```python
from build123d import *

# Parameters (mm, degrees)
MOUNT_BASE_DEPTH               = 10
SKETCH_8_W                     = 38
SKETCH_8_H                     = 31
CUT_BASE_DEPTH                 = 34
SKETCH10_W                     = 3
SKETCH10_H                     = 31
BEND_SIDES_DEPTH               = 34.2
SKETCH16_W                     = 44
SKETCH16_H                     = 3
WIRE_SIDES_DEPTH               = 34.2
DRAFT9_ANGLE                   = 1
DRAFT10_ANGLE                  = 1
DIFFERENTIAL_CLAMP_DEPTH       = 10
DIFFERENTIAL_CLAMP_DEPTH_BACK  = 8.6
DIFFERENTIAL_BAR_CUT_DEPTH     = 3.6
STRUCTURAL_SCREW_W_HEADS_DEPTH = 5
SKETCH25_R                     = 1.7
SCREW_HOLES_DEPTH              = 24
NUT_HOLE_DEPTH                 = 2.6
FILLET7_R                      = 2
FILLET8_R                      = 2
FILLET9_R                      = 2
FILLET10_R                     = 2
FILLET15_R                     = 2
BOSS_EXTRUDE1_DEPTH            = 17.6
CUT_EXTRUDE6_DEPTH             = 8.6
SKETCH48_W                     = 74
SKETCH48_H                     = 70
CUT_EXTRUDE9_DEPTH             = 17.6
SKETCH49_W                     = 77
SKETCH49_H                     = 70
BOSS_EXTRUDE2_DEPTH            = 1
SKETCH50_R                     = 1.7
CUT_EXTRUDE10_DEPTH            = 1
CUT_EXTRUDE12_DEPTH            = 34.2
SKETCH53_W                     = 19
SKETCH53_H                     = 5.77151387
CUT_EXTRUDE13_DEPTH            = 30
FILLET17_R                     = 2
BOSS_EXTRUDE3_DEPTH            = 34.2
CUT_EXTRUDE14_DEPTH            = 2.6
SKETCH56_R                     = 1.7
CUT_EXTRUDE15_DEPTH            = 8
FILLET18_R                     = 2
FILLET20_R                     = 0.5


with BuildPart() as part:
    # Sketch6 → Mount Base (new body)
    with BuildSketch(Plane(origin=(0, 0, 0), x_dir=(0, 1, 0), z_dir=(0, 0, 1))):
        Polygon((-30, -26.5), (-30, -31.5), (30, -31.5), (30, -26.5), (30, 26.5), (-30, 26.5), align=None)
    extrude(amount=MOUNT_BASE_DEPTH)

    # Sketch 8 → Cut-Base (cut)
    with BuildSketch(Plane(origin=(0, 0, 7), x_dir=(0, 1, 0), z_dir=(0, 0, 1))):
        Rectangle(SKETCH_8_W, SKETCH_8_H)
    extrude(amount=CUT_BASE_DEPTH, mode=Mode.SUBTRACT)

    # Sketch10 → Bend Sides (add)
    with BuildSketch(Plane(origin=(0, 0, 10), x_dir=(0, 1, 0), z_dir=(0, 0, 1))):
        with Locations((-20.5, 0)):
            Rectangle(SKETCH10_W, SKETCH10_H)
        with Locations((20.5, 0)):
            Rectangle(SKETCH10_W, SKETCH10_H)
    extrude(amount=BEND_SIDES_DEPTH)

    # Sketch16 → Wire Sides (add)
    with BuildSketch(Plane(origin=(0, 0, 10), x_dir=(0, 1, 0), z_dir=(0, 0, 1))):
        with Locations((0, -17)):
            Rectangle(SKETCH16_W, SKETCH16_H)
        with Locations((0, 17)):
            Rectangle(SKETCH16_W, SKETCH16_H)
    extrude(amount=WIRE_SIDES_DEPTH)

    # Draft9
    draft9_faces = [part.faces().sort_by_distance(p)[0] for p in [
        (0, -19, 25.6),
    ]]
    draft(draft9_faces, Plane(origin=(0, 0, 0), x_dir=(-1, 0, 0), z_dir=(0, 0, -1)), DRAFT9_ANGLE)

    # Draft10
    draft10_faces = [part.faces().sort_by_distance(p)[0] for p in [
        (0, 19, 25.6),
    ]]
    draft(draft10_faces, Plane(origin=(0, 0, 0), x_dir=(-1, 0, 0), z_dir=(0, 0, -1)), DRAFT10_ANGLE)

    # Sketch20 → Differential Clamp (add, two sides)
    with BuildSketch(Plane(origin=(0, 0, 0), x_dir=(0, 1, 0), z_dir=(0, 0, 1))) as differential_clamp_sk:
        Polygon((-30, 37), (-30, 26.5), (-30, -37), (30, -37), (30, 27), (30, 37), align=None)
    extrude(amount=DIFFERENTIAL_CLAMP_DEPTH)
    extrude(differential_clamp_sk.sketch, amount=-DIFFERENTIAL_CLAMP_DEPTH_BACK)

    # Sketch22 → Differential Bar cut (cut)
    with BuildSketch(Plane(origin=(0, 0, 0), x_dir=(0, 1, 0), z_dir=(0, 0, 1))):
        Polygon((-86.956180584, -24.693764348), (0, -30.5), (86.956180584, -24.693764348), (86.956180584, 37), (30, 37), (-30, 37), (-86.956180584, 37), align=None)
    extrude(amount=-DIFFERENTIAL_BAR_CUT_DEPTH, mode=Mode.SUBTRACT)

    # Sketch 7 → Structural Screw w/ heads (cut)
    with BuildSketch(Plane(origin=(0, 0, 0), x_dir=(0, 1, 0), z_dir=(0, 0, 1))):
        with BuildLine():
            Line((-22.42, 37.163783556), (-22.42, -19.42))
            ThreePointArc((-22.42, -19.42), (-19.42, -22.42), (-16.42, -19.42))
            Line((-16.42, -19.42), (-16.42, 37.163783556))
            Line((-16.42, 37.163783556), (-22.42, 37.163783556))
        make_face()
        with BuildLine():
            Line((16.42, -19.42), (16.42, 37.161181528))
            Line((16.42, 37.161181528), (22.42, 37.161181528))
            Line((22.42, 37.161181528), (22.42, -19.42))
            ThreePointArc((22.42, -19.42), (19.42, -22.42), (16.42, -19.42))
        make_face()
        with BuildLine():
            Line((-3, 37.161181528), (3, 37.161181528))
            Line((3, 37.161181528), (3, -10.32))
            ThreePointArc((3, -10.32), (0, -13.32), (-3, -10.32))
            Line((-3, -10.32), (-3, 37.161181528))
        make_face()
    extrude(amount=STRUCTURAL_SCREW_W_HEADS_DEPTH, mode=Mode.SUBTRACT)

    # Sketch25 → Screw holes (cut)
    with BuildSketch(Plane.XY.offset(10)):
        with Locations((-32, 29)):
            Circle(SKETCH25_R)
        with Locations((-32, -29)):
            Circle(SKETCH25_R)
        with Locations((32, -29)):
            Circle(SKETCH25_R)
        with Locations((32, 29)):
            Circle(SKETCH25_R)
    extrude(amount=-SCREW_HOLES_DEPTH, mode=Mode.SUBTRACT)

    # Sketch27 → Nut hole (cut)
    with BuildSketch(Plane(origin=(0, 0, -8.6), x_dir=(-1, 0, 0), z_dir=(0, 0, -1))):
        Polygon((31.935113153, 25.709743217), (34.817002535, 27.29867795), (34.881889383, 30.588934733), (32.064886847, 32.290256783), (29.182997465, 30.70132205), (29.118110617, 27.411065267), align=None)
        Polygon((28.709103466, -29), (30.354551733, -31.85), (33.645448267, -31.85), (35.290896534, -29), (33.645448267, -26.15), (30.354551733, -26.15), align=None)
        Polygon((-30.354551733, -26.15), (-28.709103466, -29), (-30.354551733, -31.85), (-33.645448267, -31.85), (-35.290896534, -29), (-33.645448267, -26.15), align=None)
        Polygon((-29.118110617, 27.411065267), (-31.935113153, 25.709743217), (-34.817002535, 27.29867795), (-34.881889383, 30.588934733), (-32.064886847, 32.290256783), (-29.182997465, 30.70132205), align=None)
    extrude(amount=-NUT_HOLE_DEPTH, mode=Mode.SUBTRACT)

    # Fillet7
    fillet7_edges = [part.edges().sort_by_distance(p)[0] for p in [
        (-37, 30, 5),
    ]]
    fillet(fillet7_edges, radius=FILLET7_R)

    # Fillet8
    fillet8_edges = [part.edges().sort_by_distance(p)[0] for p in [
        (-37, -30, 5),
    ]]
    fillet(fillet8_edges, radius=FILLET8_R)

    # Fillet9
    fillet9_edges = [part.edges().sort_by_distance(p)[0] for p in [
        (-37, 30, -6.1),
    ]]
    fillet(fillet9_edges, radius=FILLET9_R)

    # Fillet10
    fillet10_edges = [part.edges().sort_by_distance(p)[0] for p in [
        (-37, -30, -6.1),
    ]]
    fillet(fillet10_edges, radius=FILLET10_R)

    # Fillet15
    fillet15_edges = [part.edges().sort_by_distance(p)[0] for p in [
        (0, 18.825449351, 10),
        (0, -18.825449351, 10),
    ]]
    fillet(fillet15_edges, radius=FILLET15_R)

    # Sketch42 → Boss-Extrude1 (add)
    with BuildSketch(Plane.XY.offset(-8.6)):
        Polygon((37, 35), (-37, 35), (-37, 23), (28.5, 23), (28.5, -23), (-37, -23), (-37, -35), (37, -35), align=None)
    extrude(amount=BOSS_EXTRUDE1_DEPTH)

    # Sketch43 → Cut-Extrude6 (cut)
    with BuildSketch(Plane(origin=(0, 0, 0), x_dir=(-1, 0, 0), z_dir=(0, 0, -1))):
        Polygon((-24.693764348, 86.956180584), (37, 86.956180584), (37, -86.956180584), (-24.693764348, -86.956180584), (-30.5, 0), align=None)
    extrude(amount=CUT_EXTRUDE6_DEPTH, mode=Mode.SUBTRACT)

    # Sketch48 → Cut-Extrude9 (cut)
    with BuildSketch(Plane.XY.offset(9)):
        Rectangle(SKETCH48_W, SKETCH48_H)
    extrude(amount=-CUT_EXTRUDE9_DEPTH, mode=Mode.SUBTRACT)

    # Sketch49 → Boss-Extrude2 (add)
    with BuildSketch(Plane.XY.offset(9)):
        Rectangle(SKETCH49_W, SKETCH49_H)
    extrude(amount=BOSS_EXTRUDE2_DEPTH)

    # Sketch50 → Cut-Extrude10 (cut)
    with BuildSketch(Plane.XY.offset(9)):
        with Locations((-32.5, 29)):
            Circle(SKETCH50_R)
        with Locations((34.25, 29)):
            Circle(SKETCH50_R)
        with Locations((34.25, -29)):
            Circle(SKETCH50_R)
        with Locations((-32.5, -29)):
            Circle(SKETCH50_R)
    extrude(amount=CUT_EXTRUDE10_DEPTH, mode=Mode.SUBTRACT)

    # Sketch52 → Cut-Extrude12 (cut)
    with BuildSketch(Plane.XY.offset(44.2)):
        Polygon((-15.5, 24.22848613), (-9.5, 24.22848613), (-9.5, 18.22848613), (-9.5, 16.790234565), (-15.5, 16.790234565), (-15.5, 18.22848613), align=None)
        Polygon((15.5, 18.22848613), (15.5, 16.790234565), (9.5, 16.790234565), (9.5, 18.22848613), (9.5, 24.22848613), (15.5, 24.22848613), align=None)
        Polygon((15.5, -18.22848613), (15.5, -24.22848613), (9.5, -24.22848613), (9.5, -18.22848613), (9.5, -16.790234565), (15.5, -16.790234565), align=None)
        Polygon((-15.5, -18.22848613), (-15.5, -16.790234565), (-9.5, -16.790234565), (-9.5, -18.22848613), (-9.5, -24.22848613), (-15.5, -24.22848613), align=None)
    extrude(amount=-CUT_EXTRUDE12_DEPTH, mode=Mode.SUBTRACT)

    # Sketch53 → Cut-Extrude13 (cut)
    with BuildSketch(Plane.XY.offset(44.2)):
        with Locations((0, -21.114243065)):
            Rectangle(SKETCH53_W, SKETCH53_H)
        with Locations((0, 19.114243065)):
            Rectangle(SKETCH53_W, SKETCH53_H)
    extrude(amount=-CUT_EXTRUDE13_DEPTH, mode=Mode.SUBTRACT)

    # Fillet17
    fillet17_edges = [part.edges().sort_by_distance(p)[0] for p in [
        (-9.5, -20.376069039, 14.2),
    ]]
    fillet(fillet17_edges, radius=FILLET17_R)

    # Sketch55 → Boss-Extrude3 (add)
    with BuildSketch(Plane.XY.offset(10)):
        Polygon((-18.5, 22), (-18.5, -22), (-15.5, -22), (-15.5, -25), (-27.5, -25), (-27.5, -22), (-27.5, 22), (-27.5, 25), (-15.5, 25), (-15.5, 22), align=None)
        Polygon((18.5, 22), (18.5, -22), (15.5, -22), (15.5, -25), (27.5, -25), (27.5, -22), (27.5, 22), (27.5, 25), (15.5, 25), (15.5, 22), align=None)
    extrude(amount=BOSS_EXTRUDE3_DEPTH)

    # Sketch54 → Cut-Extrude14 (cut)
    with BuildSketch(Plane.XY.offset(39.2)):
        Polygon((24.4, 20.359315781), (24.4, 17.010684219), (21.5, 15.336368439), (18.6, 17.010684219), (18.6, 20.359315781), (21.5, 22.033631561), align=None)
        Polygon((-24.4, 17.010684219), (-21.5, 15.336368439), (-18.6, 17.010684219), (-18.6, 20.359315781), (-21.5, 22.033631561), (-24.4, 20.359315781), align=None)
        Polygon((21.5, -22.033631561), (24.4, -20.359315781), (24.4, -17.010684219), (21.5, -15.336368439), (18.6, -17.010684219), (18.6, -20.359315781), align=None)
        Polygon((-24.4, -20.359315781), (-24.4, -17.010684219), (-21.5, -15.336368439), (-18.6, -17.010684219), (-18.6, -20.359315781), (-21.5, -22.033631561), align=None)
    extrude(amount=CUT_EXTRUDE14_DEPTH, mode=Mode.SUBTRACT)

    # Sketch56 → Cut-Extrude15 (cut)
    with BuildSketch(Plane.XY.offset(44.2)):
        with Locations((-21.5, 18.685)):
            Circle(SKETCH56_R)
        with Locations((21.5, 18.685)):
            Circle(SKETCH56_R)
        with Locations((21.5, -18.685)):
            Circle(SKETCH56_R)
        with Locations((-21.5, -18.685)):
            Circle(SKETCH56_R)
    extrude(amount=-CUT_EXTRUDE15_DEPTH, mode=Mode.SUBTRACT)

    # Fillet18
    fillet18_edges = [part.edges().sort_by_distance(p)[0] for p in [
        (9.5, -20.376069039, 14.2),
        (-9.5, 20.376069039, 14.2),
        (9.5, 20.376069039, 14.2),
        (-21.5, 25, 44.2),
        (-21.5, -25, 44.2),
        (21.5, -25, 44.2),
        (21.5, 25, 44.2),
    ]]
    fillet(fillet18_edges, radius=FILLET18_R)

    # Fillet20
    fillet20_edges = [part.edges().sort_by_distance(p)[0] for p in [
        (-27.5, 0, 44.2),
        (-27.5, -25, 26.1),
        (-27.5, 25, 26.1),
        (-27.5, -24.414213562, 43.614213562),
        (-27.5, 24.414213562, 43.614213562),
        (-15.5, 25, 26.1),
        (-15.5, -25, 26.1),
        (-15.5, -24.414213562, 43.614213562),
        (-15.5, 24.414213562, 43.614213562),
        (15.5, 0, 44.2),
        (27.5, 0, 44.2),
        (27.5, 25, 26.1),
        (27.5, -25, 26.1),
        (27.5, 24.414213562, 43.614213562),
        (27.5, -24.414213562, 43.614213562),
        (15.5, -25, 26.1),
        (15.5, 25, 26.1),
        (15.5, 24.414213562, 43.614213562),
        (15.5, -24.414213562, 43.614213562),
        (-15.5, 0, 44.2),
    ]]
    fillet(fillet20_edges, radius=FILLET20_R)


solid = part.part
```
Design review of the part built by this model. Coordinates are the model's own, in mm. A direction names the side the tool comes from. Round coordinates to 2 decimals unless told otherwise and drop trailing zeros. Order: outer loops, then holes, each group sorted by start corner. A loop starts at its lowest first (then second) coordinate and runs counter-clockwise, first axis right, second up. Notation, with made-up numbers: (52.5, 49) - (75.5, 49) arc R22 ccw to (75.5, 83) - close; hole circle Ø5 at (13.25, 53). An arc over 180 degrees is marked (long way). Return JSON: item names as keys, results as strings.
Q1. Consider section C-C on y = 11.5. Write out the cut boundary in (x, z).
Computed values:
{"outline": "(-38.5, 9) - (38.5, 9) - (38.5, 10) - (27.5, 10) - (27.5, 43.7) arc R0.5 ccw to (27, 44.2) - (16, 44.2) arc R0.5 ccw to (15.5, 43.7) - (15.5, 10) - (-15.5, 10) - (-15.5, 43.7) arc R0.5 ccw to (-16, 44.2) - (-27, 44.2) arc R0.5 ccw to (-27.5, 43.7) - (-27.5, 10) - (-38.5, 10) - close"}
Q2. For pin 1 Ø3 at (y, z) = (18, 40.5) entering from -X; pin 2 Ø3 at (x, z) = (17.5, 30) entering from -Y; pin 3 Ø1.6 at (x, y) = (-0.5, 21) entering from +Z, all flat-tipped, find the tip position at first contact; note any pin that passes through.
Computed values:
{"pin 1": "stops at x = -27.5", "pin 2": "stops at y = -25", "pin 3": "stops at z = 14.2"}
Q3. Machinability: for faces 4 (the flat face through (-9.5, 20, 11)), 5 (the flat face through (22.93, -21.21, 40.48)), 6 (the flat face through (-22, 19, 36.2)), which of the approach directions +Z, -Z, +X, -X, +Y, -Y give a long, thin tool a straight path to every point of the face, cutting with its end or side? Answer none if there is none.
Computed values:
{"face 4": "+Z, +Y, -Y", "face 5": "none", "face 6": "+Z"}
Q4. Consider section A-A on y = 29. Write out the cut boundary in (x, z).
Computed values:
{"outline": "(-38.5, 9) - (-34.2, 9) - (-34.2, 10) - (-38.5, 10) - close; (-30.8, 9) - (32.55, 9) - (32.55, 10) - (-30.8, 10) - close; (35.95, 9) - (38.5, 9) - (38.5, 10) - (35.95, 10) - close"}
Q5. Consider section B-B on z = 17. Write out the cut boundary in (x, y).
Computed values:
{"outline": "(-27.5, -24.5) arc R0.5 ccw to (-27, -25) - (-16, -25) arc R0.5 ccw to (-15.5, -24.5) - (-15.5, 24.5) arc R0.5 ccw to (-16, 25) - (-27, 25) arc R0.5 ccw to (-27.5, 24.5) - close; (15.5, -24.5) arc R0.5 ccw to (16, -25) - (27, -25) arc R0.5 ccw to (27.5, -24.5) - (27.5, 24.5) arc R0.5 ccw to (27, 25) - (16, 25) arc R0.5 ccw to (15.5, 24.5) - close"}
Q6. Consider section D-D on z = 11. Write out the cut boundary in (x, y), plus the area to 3 significant figures.
Computed values:
{"outline": "(-27.5, -24.5) arc R0.5 ccw to (-27, -25) - (-16, -25) arc R0.5 ccw to (-15.5, -24.5) - (-15.5, 24.5) arc R0.5 ccw to (-16, 25) - (-27, 25) arc R0.5 ccw to (-27.5, 24.5) - close; (-9.5, -22) - (9.5, -22) - (9.5, -18.52) - (-9.5, -18.52) - close; (-9.5, 18.52) - (9.5, 18.52) - (9.5, 22) - (-9.5, 22) - close; (15.5, -24.5) arc R0.5 ccw to (16, -25) - (27, -25) arc R0.5 ccw to (27.5, -24.5) - (27.5, 24.5) arc R0.5 ccw to (27, 25) - (16, 25) arc R0.5 ccw to (15.5, 24.5) - close", "area": "1,330 mm2"}
Q7. Wall thickness on L1, parallel to Y at x = -21.5, z = 38.65 (3 decimals); L2, parallel to Y at x = 21, z = 43; L3, parallel to X at y = 24, z = 41: over which ranges is each line inside the solid? List them lowest first. Write a range as [from, to].
Computed values:
{"L1": "y = [-25, -20.385], [-16.985, 16.985], [20.385, 25]", "L2": "y = [-24.83, -20.31], [-17.06, 17.06], [20.31, 24.83]", "L3": "x = [-27.5, -15.5], [15.5, 27.5]"}
Q8. The part is to be moulded in two halves that separate along Y. For faces 1 (the flat face through (-20.07, -16.16, 40.48)), 2 (the flat face through (0, 22, 12)), 3 (the flat face through (-21, -25, 26)), say which applies: pulls with the +Y half, pulls with the -Y half, needs draft (parallel to the pull), parting line crosses it, or undercut.
Computed values:
{"face 1": "undercut", "face 2": "pulls with the +Y half", "face 3": "pulls with the -Y half"}
